from build123d import *

# Parameters (mm, degrees)
SKETCH6_W           = 20
SKETCH6_H           = 22
BOSS_EXTRUDE5_DEPTH = 6
SKETCH7_W           = 10
SKETCH7_H           = 22
BOSS_EXTRUDE6_DEPTH = 8
SKETCH8_W           = 14.5
SKETCH8_H           = 22
BOSS_EXTRUDE7_DEPTH = 13
SKETCH9_R           = 5
CUT_EXTRUDE1_DEPTH  = 36.284557529
FILLET1_R           = 7.5
FILLET2_R           = 7.5


with BuildPart() as part:
    # Sketch6 → Boss-Extrude5 (new body)
    with BuildSketch(Plane(origin=(0, 0, 0), x_dir=(1, 0, 0), z_dir=(0, 1, 0))):
        with Locations((10, 11)):
            Rectangle(SKETCH6_W, SKETCH6_H)
    extrude(amount=BOSS_EXTRUDE5_DEPTH)

    # Sketch7 → Boss-Extrude6 (add)
    with BuildSketch(Plane.XZ):
        with Locations((10, -11)):
            Rectangle(SKETCH7_W, SKETCH7_H)
    extrude(amount=BOSS_EXTRUDE6_DEPTH)

    # Sketch8 → Boss-Extrude7 (add)
    with BuildSketch(Plane(origin=(0, 6, 0), x_dir=(1, 0, 0), z_dir=(0, 1, 0))):
        with Locations((10, 11)):
            Rectangle(SKETCH8_W, SKETCH8_H)
    extrude(amount=BOSS_EXTRUDE7_DEPTH)

    # Sketch9 → Cut-Extrude1 (cut, through all)
    with BuildSketch(Plane.XY):
        with Locations((10, 11)):
            Circle(SKETCH9_R)
    extrude(amount=-CUT_EXTRUDE1_DEPTH, mode=Mode.SUBTRACT)

    # Fillet1
    # the kernel refuses this fillet: 7.5 mm, written as the material it takes off along each edge
    with BuildSketch(Plane(origin=(17.25, 19, -40.75), x_dir=(-1, 0, 0), z_dir=(0, 0, 1))) as fillet1_piece_1:
        with BuildLine():
            CenterArc((FILLET1_R, FILLET1_R), FILLET1_R, 180, 90)
            Line((0, FILLET1_R), (0, 0))
            Line((0, 0), (FILLET1_R, 0))
        make_face()
    extrude(amount=59.5, mode=Mode.SUBTRACT)
    with BuildSketch(Plane(origin=(2.75, 19, 18.75), x_dir=(0, -1, 0), z_dir=(0, 0, -1))) as fillet1_piece_2:
        with BuildLine():
            CenterArc((FILLET1_R, -FILLET1_R), FILLET1_R, 90, 90)
            Line((0, -FILLET1_R), (0, 0))
            Line((0, 0), (FILLET1_R, 0))
        make_face()
    extrude(amount=59.5, mode=Mode.SUBTRACT)

    # Fillet2
    # the kernel refuses this fillet: 7.5 mm, written as the material it adds along each edge
    with BuildSketch(Plane(origin=(17.25, 6, -22), x_dir=(1, 0, 0), z_dir=(0, 0, 1))) as fillet2_piece_1:
        with BuildLine():
            CenterArc((7.496865043, 5.806657581), FILLET2_R, 181.171427285, 49.563032728)
            Line((-0.001567478, 5.65332879), (-0.75141073, 5.637995911))
            ThreePointArc((-0.75141073, 5.637995911), (-0.75, 5.5), (-0.75, 0))
            Line((-0.75, 0), (0, -0.75))
            ThreePointArc((0, -0.75), (1.375, -0.75), (2.275313496, -0.580665758))
            Line((2.275313496, -0.580665758), (2.75, 0))
        make_face()
    extrude(amount=22)
    with BuildSketch(Plane(origin=(2.75, 6, 0), x_dir=(0.00027726642617420565, 0.9999999615616638, 0), z_dir=(0, 0, -1))) as fillet2_piece_2:
        with BuildLine():
            CenterArc((5.804578729, -7.498474746), FILLET2_R, 91.155541089, 49.563032728)
            Line((-0.000762483, -2.749999894), (-0.581296604, -2.275152409))
            ThreePointArc((-0.581296604, -2.275152409), (-0.750381213, -1.374791997), (-0.749999971, 0.00020795))
            Line((-0.749999971, 0.00020795), (0.00020795, 0.749999971))
            ThreePointArc((0.00020795, 0.749999971), (5.500207738, 0.748475006), (5.638204036, 0.749847475))
            Line((5.638204036, 0.749847475), (5.653329008, 0))
        make_face()
    extrude(amount=22)


solid = part.part
Input: part model. Units: mm. Frame: model coordinates. A direction names the side the tool comes from. Give positions to 0.01 mm unless a question says otherwise; leave off trailing zeros. Order: outer loops, then holes, each group sorted by start corner. A loop starts at its lowest first (then second) coordinate and runs counter-clockwise, first axis right, second up. Notation, with made-up numbers: (66.25, 35.25) - (112.25, 35.25) arc R22 cw to (112.25, 61.25) - close; hole circle Ø3 at (34, 74). An arc over 180 degrees is marked (long way). Answer as a JSON object with one key per item and string values. Group by question number.
Q1. Cut plane C-C, the plane y = 11. Output: boundary loops of the cut face in (x, z).
Q2. Line query: probe 1 along Y at (x, z) = (10, -13.25); probe 2 along X at (y, z) = (-3.25, -4); probe 3 along Y at (x, z) = (9.25, -12.5). Output: solid intervals per line, ascending.
Q3. Cut plane A-A, the plane x = 12.5. Output: boundary loops of the cut face in (y, z).
Q4. First-contact query: pin 1 Ø4 at (x, z) = (2, -6.5) entering from -Y; pin 2 Ø11.5 at (x, y) = (10, 11) entering from +Z; pin 3 Ø6.5 at (y, z) = (-5.5, -13) entering from -X; pin 4 Ø1 at (y, z) = (12.5, -3) entering from -X. Flat tips, straight axial feed; report the tip coordinate or a pass-through.
Q5. Cut plane D-D, the plane y = 17.5. Output: boundary loops of the cut face in (x, z).
Q6. Set-up query: faces 1 (the face through (5, -4, -11)), 2 (the face through (10, 3, 0)), 3 (the face through (17, 0, -11)). Return all of +Z, -Z, +X, -X, +Y, -Y with unobstructed straight access to the full face (end or side cutting, diameter ignored); none if empty.
Q7. Mould query, pull axis X, two halves, no side actions, for faces 4 (the face through (14.77, 12.5, -10.85)), 5 (the face through (10, 3, -22)), 6 (the face through (0, 3, -11)). Classes: pulls with the +X half, pulls with the -X half, needs draft (parallel to the pull), parting line crosses it, or undercut.
Q8. Cut plane B-B, the plane z = -4.5. Output: boundary loops of the cut face in (x, y).
Results:
{
 "1": {"outline": "(2.71, -22) - (5, -22) - (5, 0) - (2.71, 0) - close; (15, -22) - (17.29, -22) - (17.29, 0) - (15, 0) - close"},
 "2": {"probe 1": "-8 to 6, 16 to 19", "probe 2": "5 to 15", "probe 3": "-8 to 6.06, 15.94 to 18.93"},
 "3": {"outline": "(-8, -22) - (6.67, -22) - (6.67, 0) - (-8, 0) - close; (15.33, -22) - (18.48, -22) - (18.48, 0) - (15.33, 0) - close"},
 "4": {"pin 1": "y = 0", "pin 2": "z = 0", "pin 3": "x = 5", "pin 4": "x = 2.77"},
 "5": {"outline": "(5.75, -22) - (14.25, -22) - (14.25, 0) - (5.75, 0) - close"},
 "6": {"face 1": "+Z, -Z, -X, -Y", "face 2": "+Z, +X, -X, +Y, -Y", "face 3": "+Z, -Z, +X, -Y"},
 "7": {"face 4": "undercut", "face 5": "needs draft", "face 6": "pulls with the -X half"},
 "8": {"outline": "(0, 0) - (5, 0) - (5, -8) - (15, -8) - (15, 0) - (20, 0) - (20, 6) arc R7.5 cw to (17.25, 11.65) arc R7.5 ccw to (10, 19) arc R7.5 ccw to (2.75, 11.65) arc R7.5 cw to (0, 6) - close; hole circle Ø10 at (10, 11)"}
}
